The drawing under review shows one solid part. Ordinate dimensions are in mm from its lowest x, y, z. A direction names the side the tool comes from. Round coordinates to 2 decimals unless told otherwise and drop trailing zeros. Order: outer loops, then holes, each group sorted by start corner. A loop starts at its lowest first (then second) coordinate and runs counter-clockwise, first axis right, second up. Notation, with made-up numbers: (83.5, 26.5) -> (134.5, 26.5) arc R10 cw to (134.5, 30.5) -> close; hole circle Ø2 at (70.25, 86.25). An arc over 180 degrees is marked (long way). Use a Markdown table: item, result. Add a question column.
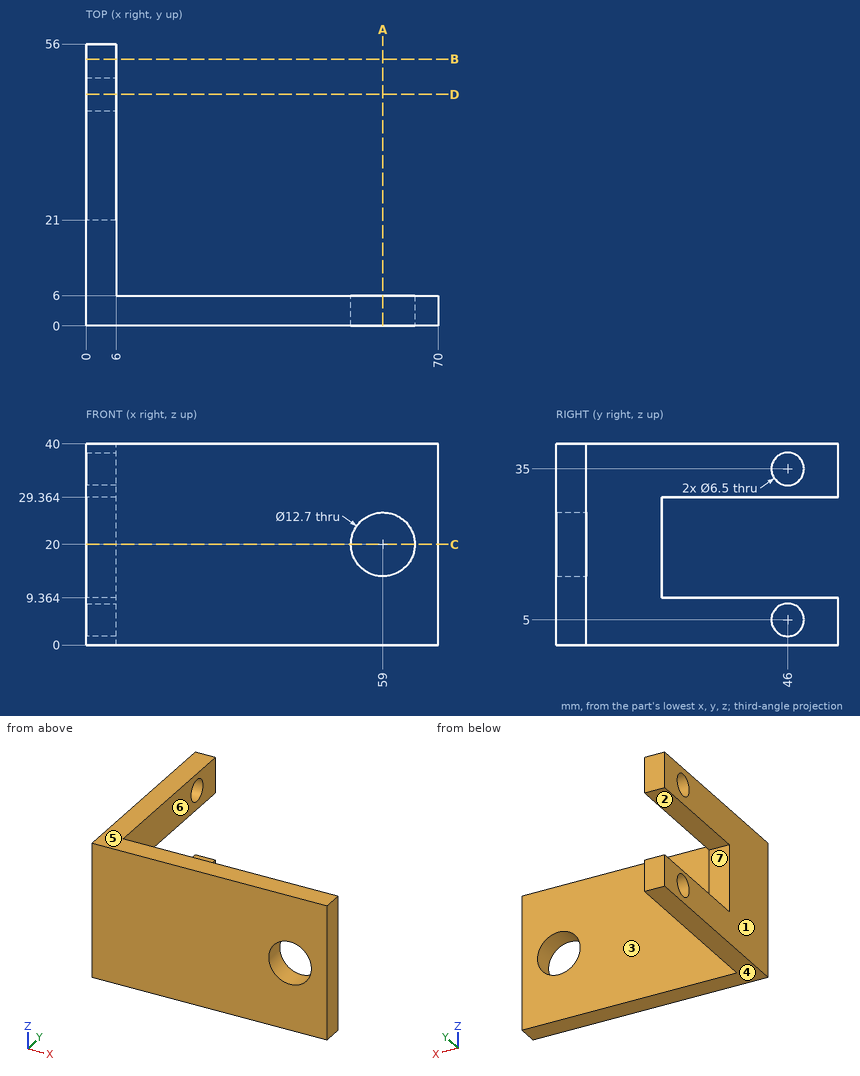
Q1. For the marked faces 1, 2 and 3, list the 3-axis set-ups (+Z, -Z, +X, -X, +Y, -Y) from which the entire face can be reached by the end or side of a thin tool; tool diameter is ignored.
Q2. Add section A-A, the plane x = 59. Give the boundary of the cut face in (y, z).
Q3. Add section D-D, the plane y = 46. Give the boundary of the cut face in (x, z), then the cut area to 3 significant figures.
Q4. Add section B-B, the plane y = 53. Give the boundary of the cut face in (x, z), then the cut area to 3 significant figures.
Q5. Draft analysis for pull direction Z (two halves, no side actions). For the marked faces 4, 5, 6 and 7, state which applies: released by +Z, released by -Z, zero draft, split by the parting line, or undercut.
Q6. Add section C-C, the plane z = 20. Give the boundary of the cut face in (x, y), then the cut area to 3 significant figures.
Q7. For pin 1 (20 mm diameter, centred on x = 47, z = 28, fed in from +Y); pin 2 (20 mm diameter, centred on y = 30.5, z = 13, fed in from +X); pin 3 (3 mm diameter, centred on x = 1.5, z = 24, fed in from +Y), all flat-tipped, find the tip position at first contact; note any pin that passes through.
Q8. To check wall thickness, follow line 1 along X through (y, z) = (1, 20); line 2 along Y through (x, z) = (3, 35); line 3 along Y through (x, z) = (56, 31.5). State the ranges of each line that lie inside material, in increasing order.
Return value:
| question | item | result |
|---|---|---|
| 1 | face 1 | +Z, -Z, -X, +Y, -Y |
| 1 | face 2 | +X, -X, +Y |
| 1 | face 3 | +Z, -Z, +X, +Y |
| 2 | outline | (0, 0) -> (6, 0) -> (6, 13.65) -> (0, 13.65) -> close; (0, 26.35) -> (6, 26.35) -> (6, 40) -> (0, 40) -> close |
| 3 | outline | (0, 0) -> (6, 0) -> (6, 1.75) -> (0, 1.75) -> close; (0, 8.25) -> (6, 8.25) -> (6, 9.36) -> (0, 9.36) -> close; (0, 29.36) -> (6, 29.36) -> (6, 31.75) -> (0, 31.75) -> close; (0, 38.25) -> (6, 38.25) -> (6, 40) -> (0, 40) -> close |
| 3 | area | 42.0 mm² |
| 4 | outline | (0, 0) -> (6, 0) -> (6, 9.36) -> (0, 9.36) -> close; (0, 29.36) -> (6, 29.36) -> (6, 40) -> (0, 40) -> close |
| 4 | area | 120 mm² |
| 5 | face 4 | released by -Z |
| 5 | face 5 | released by +Z |
| 5 | face 6 | zero draft |
| 5 | face 7 | undercut |
| 6 | outline | (0, 0) -> (52.65, 0) -> (52.65, 6) -> (6, 6) -> (6, 21) -> (0, 21) -> close; (65.35, 0) -> (70, 0) -> (70, 6) -> (65.35, 6) -> close |
| 6 | area | 434 mm² |
| 7 | pin 1 | y = 6 |
| 7 | pin 2 | x = 6 |
| 7 | pin 3 | y = 21 |
| 8 | line 1 | 0 to 52.65, 65.35 to 70 |
| 8 | line 2 | 0 to 42.75, 49.25 to 56 |
| 8 | line 3 | 0 to 6 |
